Input: part model. Units: mm. Frame: model coordinates. A direction names the side the tool comes from. Give positions to 0.01 mm unless a question says otherwise; leave off trailing zeros. Order: outer loops, then holes, each group sorted by start corner. A loop starts at its lowest first (then second) coordinate and runs counter-clockwise, first axis right, second up. Notation, with made-up numbers: (40.5, 8) - (71.5, 8) arc R23 cw to (71.5, 39) - close; hole circle Ø8 at (82.25, 62.5). An arc over 180 degrees is marked (long way). Answer in a Markdown table with one row per item. Add a question column.
1. Section query C-C on z = -3. Return loops of the section in (x, y), and give its area (4 significant figures).
2. Access query for faces 1 (the face through (28, 17, -20)), 2 (the face through (27.5, 32.92, -19.92)), 3 (the face through (6.57, 17.74, -13.95)). Directions: +Z, -Z, +X, -X, +Y, -Y. A direction counts if a zero-diameter tool reaches every point of the face in a straight line with its end or side. Return the directions, or none.
3. Mould query, pull axis Z, two halves, no side actions, for faces 4 (the face through (-1, 0, -11)), 5 (the face through (-6.55, 17.74, -11.83)), 6 (the face through (33.309, -2.465, -2.146)), 7 (the face through (-36.756, -2.465, -3.401)). Classes: released by +Z, released by -Z, zero draft, split by the parting line, or undercut.
4. Section query B-B on y = 4. Count the separate pieces of the cut face and the enclosed holes in it, and give its area (3 significant figures).
5. Contact query for flat-ended pins moving along their axis: pin 1 (1.5 mm diameter, centred on x = -2, y = 30, fed in from -Z); pin 2 (3.5 mm diameter, centred on y = 13, z = -19.5, fed in from +X); pin 3 (2 mm diameter, centred on x = 25, y = 22.5, fed in from +Z). Output: stop coordinate, or through.
6. Section query A-A on x = 25.75. Return loops of the section in (y, z).
7. Ray query, line 1 (Y direction, x = 25.75, z = -19.4); line 2 (X direction, y = -3.4, z = -3); line 3 (X direction, y = 4, z = -19.6). Return the intervals inside material, ascending. Write a range as [from, to].
```python
from build123d import *

# Parameters (mm, degrees)
SKETCH_1_R          = 1.85
EXTRUDE_1_DEPTH     = 5
SKETCH_2_W          = 4.5
SKETCH_2_H          = 3
SKETCH_2_W_2        = 14
EXTRUDE_2_DEPTH     = 35
SKETCH_4_R          = 1.75
CUT_EXTRUDE_2_DEPTH = 35
FILLET_3_R          = 1.5
FILLET_4_R          = 1.5


with BuildPart() as part:
    # 草图1 → 凸台-拉伸1 (new body)
    with BuildSketch(Plane(origin=(0, 0, 0), x_dir=(1, 0, 0), z_dir=(0, 1, 0))):
        Polygon((-38.55, 0), (38.55, 0), (38.55, 6), (28, 21.4), (-28, 21.4), (-38.55, 6), align=None)
        with Locations(Location((-34.95, 3, 0), (0, 0, 270))):
            Circle(SKETCH_1_R, mode=Mode.SUBTRACT)
        with Locations(Location((34.95, 3, 0), (0, 0, 270))):
            Circle(SKETCH_1_R, mode=Mode.SUBTRACT)
    extrude(amount=-EXTRUDE_1_DEPTH)

    # 草图2 → 凸台-拉伸2 (add)
    with BuildSketch(Plane(origin=(0, 0, 0), x_dir=(1, 0, 0), z_dir=(0, 1, 0))):
        with Locations((25.75, 19.9)):
            Rectangle(SKETCH_2_W, SKETCH_2_H)
        with Locations((0, 12.9)):
            Rectangle(SKETCH_2_W_2, SKETCH_2_H)
    extrude(amount=EXTRUDE_2_DEPTH)

    # 草图4 → 切除-拉伸2 (cut)
    with BuildSketch(Plane.XY.offset(-21.4)):
        with Locations(Location((25.75, 33, 0), (0, 0, 180))):
            Circle(SKETCH_4_R)
        with Locations(Location((25.75, 4, 0), (0, 0, 180))):
            Circle(SKETCH_4_R)
    extrude(amount=CUT_EXTRUDE_2_DEPTH, mode=Mode.SUBTRACT)

    # 圆角3
    fillet_3_edges = [part.edges().sort_by_distance(p)[0] for p in [
        (-7, 17.5, -14.4),
        (-7, 17.5, -11.4),
        (7, 17.5, -14.4),
        (7, 17.5, -11.4),
        (0, 35, -11.4),
        (0, 35, -14.4),
    ]]
    fillet(fillet_3_edges, radius=FILLET_3_R - 0.0001)  # a hair under: the kernel refuses the full size

    # 圆角4
    fillet_4_edges = [part.edges().sort_by_distance(p)[0] for p in [
        (-38.55, -2.5, -6),
        (-28, -2.5, -21.4),
        (38.55, -2.5, -6),
        (38.55, -2.5, 0),
        (-38.55, -2.5, 0),
    ]]
    fillet(fillet_4_edges, radius=FILLET_4_R)


solid = part.part
```
Answer:
| question | item | result |
|---|---|---|
| 1 | outline | (-38.55, -5) - (-36.8, -5) - (-36.8, 0) - (-38.55, 0) - close; (-33.1, -5) - (33.1, -5) - (33.1, 0) - (-33.1, 0) - close; (36.8, -5) - (38.55, -5) - (38.55, 0) - (36.8, 0) - close |
| 1 | area | 348.5 mm² |
| 2 | face 1 | +Z, -Z, +X, +Y |
| 2 | face 2 | +Z, -Z |
| 2 | face 3 | -Z, +X, +Y |
| 3 | face 4 | zero draft |
| 3 | face 5 | released by +Z |
| 3 | face 6 | undercut |
| 3 | face 7 | undercut |
| 4 | separate pieces | 3 |
| 4 | enclosed holes | 0 |
| 4 | area | 43.1 mm² |
| 5 | pin 1 | stops at z = -14.4 |
| 5 | pin 2 | stops at x = 28 |
| 5 | pin 3 | stops at z = -18.4 |
| 6 | outline | (-5, -21.4) - (2.25, -21.4) - (2.25, -18.4) - (0, -18.4) - (0, 0) - (-5, 0) - close; (5.75, -21.4) - (31.25, -21.4) - (31.25, -18.4) - (5.75, -18.4) - close; (34.75, -21.4) - (35, -21.4) - (35, -18.4) - (34.75, -18.4) - close |
| 7 | line 1 | y = [-5, 2.25], [5.75, 31.25], [34.75, 35] |
| 7 | line 2 | x = [-38.55, -36.8], [-33.1, 33.1], [36.8, 38.55] |
| 7 | line 3 | x = [23.5, 24], [27.5, 28] |
